```python
from build123d import *

# Parameters (mm, degrees)
SKETCH2_R          = 1
CUT_EXTRUDE1_DEPTH = 10
SKETCH3_R          = 1
CUT_EXTRUDE2_DEPTH = 10
CIRPATTERN1_COUNT  = 8
CIRPATTERN2_COUNT  = 4
SKETCH5_R          = 1.5
CUT_EXTRUDE3_DEPTH = 10


with BuildPart() as part:
    # Sketch1 → Revolve1 (revolve)
    with BuildSketch(Plane.XY, mode=Mode.PRIVATE) as revolve1_sk:
        Polygon((0, 0), (0, 4.95), (2, 4.95), (2, 13.9), (4.4, 13.9), (4.4, 0), align=None)
    revolve(revolve1_sk.sketch.rotate(Axis((0, 0, 0), (1, 0, 0)), 90), axis=Axis((0, 0, 0), (1, 0, 0)))

    # Sketch2 → Cut-Extrude1 (cut)
    with BuildSketch(Plane(origin=(4.4, 0, 0), x_dir=(0, 0, -1), z_dir=(1, 0, 0))):
        with Locations((0, 11)):
            Circle(SKETCH2_R)
    cut_extrude1 = extrude(amount=-CUT_EXTRUDE1_DEPTH, mode=Mode.SUBTRACT)

    # Sketch3 → Cut-Extrude2 (cut)
    with BuildSketch(Plane(origin=(4.4, 0, 0), x_dir=(0, 0, -1), z_dir=(1, 0, 0))):
        with Locations((0, 8.5)):
            Circle(SKETCH3_R)
    cut_extrude2 = extrude(amount=-CUT_EXTRUDE2_DEPTH, mode=Mode.SUBTRACT)

    # CirPattern1: Cut-Extrude1 ×8 about axis
    cirpattern1_axis = Axis((0, 0, 0), (1, 0, 0))
    for i in range(1, CIRPATTERN1_COUNT):
        add(cut_extrude1.rotate(cirpattern1_axis, i * 360 / CIRPATTERN1_COUNT), mode=Mode.SUBTRACT)

    # CirPattern2: Cut-Extrude2 ×4 about axis
    cirpattern2_axis = Axis((0, 0, 0), (1, 0, 0))
    for i in range(1, CIRPATTERN2_COUNT):
        add(cut_extrude2.rotate(cirpattern2_axis, i * 360 / CIRPATTERN2_COUNT), mode=Mode.SUBTRACT)

    # Sketch5 → Cut-Extrude3 (cut)
    with BuildSketch(Plane(origin=(4.4, 0, 0), x_dir=(0, 0, -1), z_dir=(1, 0, 0))):
        Circle(SKETCH5_R)
    extrude(amount=-CUT_EXTRUDE3_DEPTH, mode=Mode.SUBTRACT)


solid = part.part
```
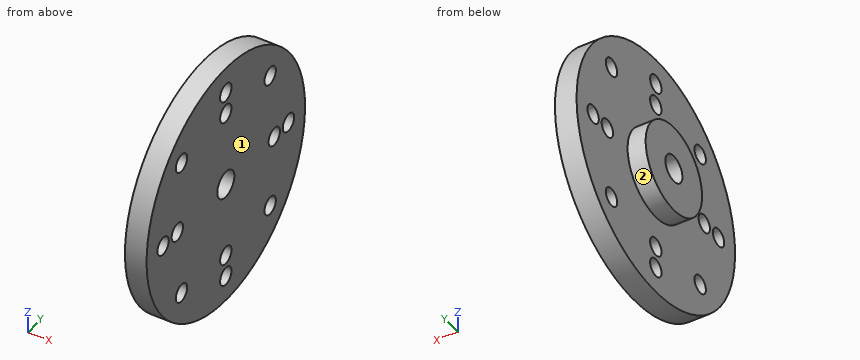
The listing builds one solid part. Answer for the finished solid, in the listing's coordinates (mm). Face numbers are marked on the shaded views. A direction names the side the tool comes from. Round coordinates to 2 decimals unless told otherwise and drop trailing zeros. Order: outer loops, then holes, each group sorted by start corner. A loop starts at its lowest first (then second) coordinate and runs counter-clockwise, first axis right, second up. Notation, with made-up numbers: (81.5, -9) -> (109.5, -9) arc R23 ccw to (109.5, 18) -> close; hole circle Ø8 at (-35, -12.5). An arc over 180 degrees is marked (long way). Answer as CSV lines item,"result".
Q1. Given pin 1 (6 mm diameter, centred on y = 3.5, z = -6.5, fed in from -X); pin 2 (2 mm diameter, centred on y = -1, z = 7, fed in from -X); pin 3 (2 mm diameter, centred on x = 4, z = 7.5, fed in from -Y), each flat-ended and moving along its own axis, determine where each tip first touches the part or whether it passes through.
Computed values:
pin 1,"stops at x = 0"
pin 2,"stops at x = 2"
pin 3,"stops at y = -12.29"
Q2. Which of the six approach directions +Z, -Z, +X, -X, +Y, -Y give full straight-line access (tool end or side, diameter ignored) to the marked faces 1 and 2?
Computed values:
face 1,"+Z, -Z, +X, +Y, -Y"
face 2,"-X"
Q3. A cutting plane is placed at C-C on y = 11. Determine the outline of the cut face in (x, z), plus the area to 3 significant figures.
Computed values:
outline,"(2, -8.5) -> (4.4, -8.5) -> (4.4, -1) -> (2, -1) -> close; (2, 1) -> (4.4, 1) -> (4.4, 8.5) -> (2, 8.5) -> close"
area,"36.0 mm^2"
Q4. A cutting plane is placed at D-D on x = 2.6. Give the number of separate pieces and of enclosed holes in the cut face, plus the area to 3 significant figures.
Computed values:
separate pieces,"1"
enclosed holes,"13"
area,"562 mm^2"
Q5. Consider line 1 (Y direction, x = 2.95, z = 0); line 2 (X direction, y = -9, z = -3); line 3 (Y direction, x = 3.7, z = -1.25). Determine where each line is inside the solid, lowest interval first. Write a range as from..to.
Computed values:
line 1,"y = -13.9..-12, -10..-9.5, -7.5..-1.5, 1.5..7.5, 9.5..10, 12..13.9"
line 2,"x = 2..4.4"
line 3,"y = -13.84..-0.83, 0.83..13.84"
Q6. A cutting plane is placed at B-B on x = 1. Determine the outline of the cut face in (y, z), plus the area to 3 significant figures.
Computed values:
outline,"circle Ø9.9 at (0, 0); hole circle Ø3 at (0, 0)"
area,"69.9 mm^2"
Q7. A cutting plane is placed at A-A on z = -11.5. Determine the outline of the cut face in (x, y), plus the area to 3 significant figures.
Computed values:
outline,"(2, -7.81) -> (4.4, -7.81) -> (4.4, -0.87) -> (2, -0.87) -> close; (2, 0.87) -> (4.4, 0.87) -> (4.4, 7.81) -> (2, 7.81) -> close"
area,"33.3 mm^2"
